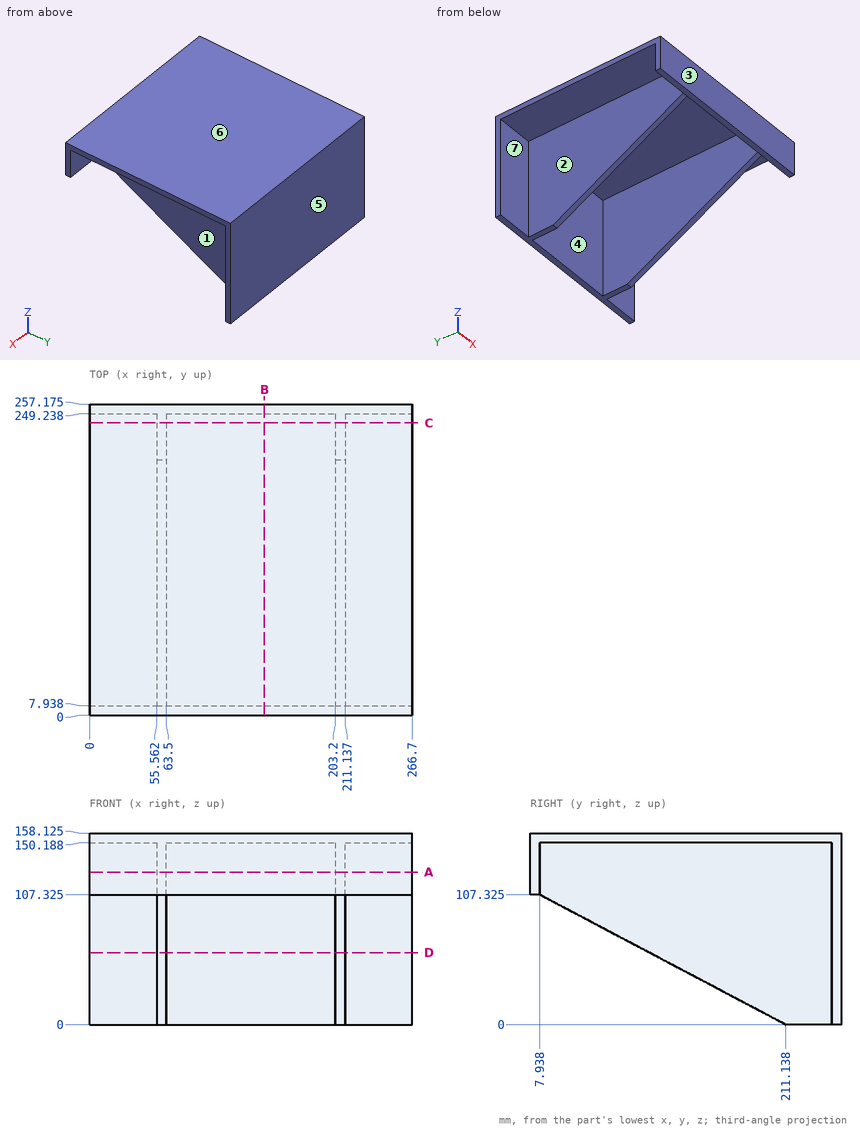
Drawing for the job (mm, zero at the part's lowest x, y, z). A direction names the side the tool comes from. Give positions to 0.01 mm unless a question says otherwise; leave off trailing zeros. Loops run counter-clockwise (first coordinate to the right, second up) from the corner with the lowest first, then second, coordinate; pieces in that order, holes last.
(1) Band-saw the part on B-B (x = 144.5). Write the cut outline in (y, z) (1 decimal).
Return value:
outline: (0, 107.3) - (7.9, 107.3) - (7.9, 150.2) - (249.2, 150.2) - (249.2, 0) - (257.2, 0) - (257.2, 158.1) - (0, 158.1) - close
(2) Pin check, flat tips, straight feed: pin 1 (1.5 mm diameter, centred on y = 166.5, z = 131.5, fed in from +X); pin 2 (16.5 mm diameter, centred on x = 241, y = 144.5, fed in from -Z); pin 3 (1 mm diameter, centred on x = 193, z = 63.5, fed in from -Y). Stop position of each tip, or through.
Return value:
pin 1: stops at x = 211.14
pin 2: stops at z = 150.19
pin 3: stops at y = 249.24
(3) Pull direction Y, two halves, no side cores. Call the marked faces 5, 6 and 7: pulls with the +Y half, pulls with the -Y half, needs draft (parallel to the pull), parting line crosses it, or undercut.
Return value:
face 5: pulls with the +Y half
face 6: needs draft
face 7: undercut
(4) Band-saw the part on A-A (z = 126). Write the cut outline in (x, y) (1 decimal).
Return value:
outline: (0, 0) - (266.7, 0) - (266.7, 7.9) - (211.1, 7.9) - (211.1, 249.2) - (266.7, 249.2) - (266.7, 257.2) - (0, 257.2) - (0, 249.2) - (55.6, 249.2) - (55.6, 7.9) - (0, 7.9) - close; hole (63.5, 7.9) - (203.2, 7.9) - (203.2, 249.2) - (63.5, 249.2) - close
(5) Drill centre lines: line 1 along X through (y, z) = (216.5, 28.5); line 2 along Y through (x, z) = (255, 115.5) (1 decimal); line 3 along Z through (x, y) = (251, 72.5) (1 decimal). Where is each one in solid material? Low to high.
Return value:
line 1: x = 55.56 to 63.5, 203.2 to 211.14
line 2: y = 0 to 7.9, 249.2 to 257.2
line 3: z = 150.2 to 158.1
(6) Band-saw the part on C-C (y = 241.5). Write the cut outline in (x, z) (1 decimal), and give its area (3 significant figures).
Return value:
outline: (0, 150.2) - (55.6, 150.2) - (55.6, 0) - (63.5, 0) - (63.5, 150.2) - (203.2, 150.2) - (203.2, 0) - (211.1, 0) - (211.1, 150.2) - (266.7, 150.2) - (266.7, 158.1) - (0, 158.1) - close
area: 4,500 mm2
(7) Band-saw the part on D-D (z = 59.5). Write the cut outline in (x, y) (1 decimal).
Return value:
outline: (0, 249.2) - (55.6, 249.2) - (55.6, 98.5) - (63.5, 98.5) - (63.5, 249.2) - (203.2, 249.2) - (203.2, 98.5) - (211.1, 98.5) - (211.1, 249.2) - (266.7, 249.2) - (266.7, 257.2) - (0, 257.2) - close
(8) 3-axis set-ups, long thin cutter, end or side, ignore diameter. For the marked faces 1, 2, 3 and 4: which of +Z, -Z, +X, -X, +Y, -Y reach the whole face in a straight line?
Return value:
face 1: -Z, +X
face 2: -Z, -X
face 3: +Z, -Z, +X, -X, -Y
face 4: -Z
